from build123d import *

# Parameters (mm, degrees)
SKETCH1_W           = 381
SKETCH1_H           = 76.2
BOSS_EXTRUDE1_DEPTH = 12.7
CUT_EXTRUDE1_REACH  = 14.7
SKETCH2_R           = 10.31875


with BuildPart() as part:
    # Sketch1 → Boss-Extrude1 (new body)
    with BuildSketch(Plane(origin=(0, 0, 0), x_dir=(1, 0, 0), z_dir=(0, 1, 0))):
        with Locations((190.5, 38.1)):
            Rectangle(SKETCH1_W, SKETCH1_H)
    extrude(amount=BOSS_EXTRUDE1_DEPTH)

    # Sketch2 → Cut-Extrude1 (cut, up to next)
    with BuildSketch(Plane(origin=(0, 12.7, 0), x_dir=(1, 0, 0), z_dir=(0, 1, 0)), mode=Mode.PRIVATE) as cut_extrude1_sk1:
        with Locations((38.1, 38.1)):
            Circle(SKETCH2_R)
    cut_extrude1_tool1 = extrude(cut_extrude1_sk1.sketch, amount=-CUT_EXTRUDE1_REACH, mode=Mode.PRIVATE) & part.part
    add(cut_extrude1_tool1.solids().sort_by_distance((38.1, 12.7, -38.1))[0], mode=Mode.SUBTRACT)
    # Sketch2 → Cut-Extrude1 (cut, up to next)
    with BuildSketch(Plane(origin=(0, 12.7, 0), x_dir=(1, 0, 0), z_dir=(0, 1, 0)), mode=Mode.PRIVATE) as cut_extrude1_sk2:
        with Locations((342.9, 38.1)):
            Circle(SKETCH2_R)
    cut_extrude1_tool2 = extrude(cut_extrude1_sk2.sketch, amount=-CUT_EXTRUDE1_REACH, mode=Mode.PRIVATE) & part.part
    add(cut_extrude1_tool2.solids().sort_by_distance((342.9, 12.7, -38.1))[0], mode=Mode.SUBTRACT)


solid = part.part
CAD build for the part. Positions are in the model's coordinates, mm. Coordinates: 2 decimals unless noted, no trailing zeros. Write each loop counter-clockwise with the first axis right and the second up, starting at its lowest first coordinate (ties: lowest second). Pieces come first, ordered by that corner, then holes. Notation, with made-up numbers: (-17, 13) - (14, 13) arc R12 cw to (14, 26) - close; hole circle Ø2 at (3, 2.5). An arc over 180 degrees is marked (long way). Use a Markdown table: item, result. Add a question column.
Item 1: Drill centre lines: L1, parallel to X at y = 4, z = -38.1; L2, parallel to Z at x = 342.9, y = 2.75. Where is each one in solid material? Low to high. Write a range as from..to.
Item 2: Band-saw the part on A-A, the plane z = -38.1. Give the cut face in (x, y), and give its area (3 significant figures).
Item 3: Band-saw the part on C-C, the plane y = 5. Give the cut face in (x, z).
Item 4: Band-saw the part on B-B, the plane x = 342.9. Give the cut face in (y, z).
Item 5: Mould opens along X. For faces 1 (the face through (47.94, 6.44, -41.2)), 2 (the face through (0, 6, -38)), 3 (the face through (332.59, 6.44, -38.55)), 4 (the face through (188, 12.7, -39)) say: pulls with the +X half, pulls with the -X half, needs draft (parallel to the pull), parting line crosses it, or undercut.
Numbers:
| question | item | result |
|---|---|---|
| 1 | L1 | 0..27.78, 48.42..332.58, 353.22..381 |
| 1 | L2 | -76.2..-48.42, -27.78..0 |
| 2 | outline | (0, 0) - (27.78, 0) - (27.78, 12.7) - (0, 12.7) - close; (48.42, 0) - (332.58, 0) - (332.58, 12.7) - (48.42, 12.7) - close; (353.22, 0) - (381, 0) - (381, 12.7) - (353.22, 12.7) - close |
| 2 | area | 4,310 mm2 |
| 3 | outline | (0, -76.2) - (381, -76.2) - (381, 0) - (0, 0) - close; hole circle Ø20.64 at (38.1, -38.1); hole circle Ø20.64 at (342.9, -38.1) |
| 4 | outline | (0, -76.2) - (12.7, -76.2) - (12.7, -48.42) - (0, -48.42) - close; (0, -27.78) - (12.7, -27.78) - (12.7, 0) - (0, 0) - close |
| 5 | face 1 | undercut |
| 5 | face 2 | pulls with the -X half |
| 5 | face 3 | undercut |
| 5 | face 4 | needs draft |
